```python
from build123d import *

# Parameters (mm, degrees)
SKETCH4_R           = 5
BOSS_EXTRUDE6_DEPTH = 15
SKETCH9_R           = 10.43494917
SKETCH9_R_2         = 5
BOSS_EXTRUDE8_DEPTH = 10.5


with BuildPart() as part:
    # Sketch4 → Boss-Extrude6 (new body)
    with BuildSketch(Plane.XY):
        with BuildLine():
            Line((101.689180826, -7.145205758), (62.319180826, -7.145205758))
            Line((62.319180826, -7.145205758), (62.319180826, 3.125413503))
            Line((62.319180826, 3.125413503), (101.689180826, 3.125413503))
            ThreePointArc((101.689180826, 3.125413503), (120.269891461, -2.009896128), (101.689180826, -7.145205758))
        make_face()
        with Locations((110.269891461, -2.009896128)):
            Circle(SKETCH4_R, mode=Mode.SUBTRACT)
    extrude(amount=BOSS_EXTRUDE6_DEPTH)

    # Sketch9 → Boss-Extrude8 (add)
    with BuildSketch(Plane(origin=(0, 3.125413503, 0), x_dir=(1, 0, 0), z_dir=(0, 1, 0))):
        with Locations(Location((55.063964483, -7.5, 0), (0, 0, 180))):
            Circle(SKETCH9_R)
        with Locations(Location((55.063964483, -7.5, 0), (0, 0, 180))):
            Circle(SKETCH9_R_2, mode=Mode.SUBTRACT)
    extrude(amount=-BOSS_EXTRUDE8_DEPTH)


solid = part.part
```
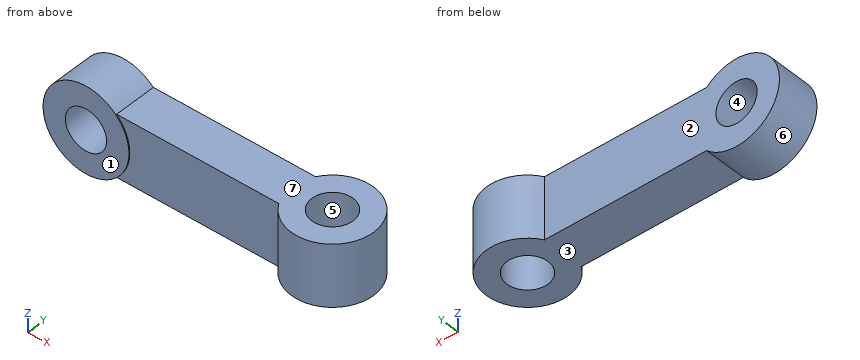
Input: part model. Units: mm. Frame: model coordinates. Face numbers are marked on the shaded views. A direction names the side the tool comes from. Round coordinates to 2 decimals unless told otherwise and drop trailing zeros. Loops run counter-clockwise (first coordinate to the right, second up) from the corner with the lowest first, then second, coordinate; pieces in that order, holes last. Notation, with made-up numbers: (-3, 23.25) - (48, 23.25) arc R11 cw to (48, 31.25) - close; hole circle Ø10 at (24, 50). An arc over 180 degrees is marked (long way). One line per item, written item: value. Start each with the question number.
(1) Section A-A, the plane z = 7.5. Return loops of the section in (x, y).
(2) Section B-B, the plane x = 107. Return loops of the section in (y, z), plus the area to 3 significant figures.
(3) Section C-C, the plane z = 13.5. Return loops of the section in (x, y), plus the area to 3 significant figures.
(4) Access query for the marked faces 1, 2 and 3. Directions: +Z, -Z, +X, -X, +Y, -Y. A direction counts if a zero-diameter tool reaches every point of the face in a straight line with its end or side. Return the directions, or none.
(5) Ray query, line 1 (X direction, y = -1, z = 5); line 2 (X direction, y = 0.5, z = 11.75); line 3 (Y direction, x = 59.5, z = -1.25). Return the intervals inside material, ascending. Write a range as [from, to].
(6) Section D-D, the plane z = 4.25. Return loops of the section in (x, y), plus the area to 3 significant figures.
(7) Draft query along Z for the marked faces 4, 5, 6 and 7. Return one class per face: +Z half, -Z half, draft (parallel to the pull), parting line (faces both ways), or undercut.
(8) Contact query for flat-ended pins moving along their axis: P1, Ø6, axis at x = 103, z = 2, coming from the +Y side; P2, Ø10, axis at y = -4.5, z = -0.5, coming from the -X side; P3, Ø1, axis at y = -4, z = 6, coming from the +X side. Output: stop coordinate, or through.
Results below:
1. outline: (44.63, -7.37) - (50.06, -7.37) - (50.06, 3.13) - (44.63, 3.13) - close; (60.06, -7.37) - (65.5, -7.37) - (65.5, -7.15) - (101.69, -7.15) arc R10 ccw (long way) to (101.69, 3.13) - (60.06, 3.13) - close; hole circle Ø10 at (110.27, -2.01)
2. outline: (-11.46, 0) - (-5.79, 0) - (-5.79, 15) - (-11.46, 15) - close; (1.77, 0) - (7.44, 0) - (7.44, 15) - (1.77, 15) - close
2. area: 170 mm^2
3. outline: (46.53, -7.37) - (63.6, -7.37) - (63.6, -7.15) - (101.69, -7.15) arc R10 ccw (long way) to (101.69, 3.13) - (46.53, 3.13) - close; hole circle Ø10 at (110.27, -2.01)
3. area: 796 mm^2
4. face 1: +Z, -Z, -X, -Y
4. face 2: +Z, -Z, -X, +Y
4. face 3: -Z, +X, +Y, -Y
5. line 1: [44.93, 50.73], [59.39, 105.37], [115.17, 120.22]
5. line 2: [45.53, 52.43], [57.7, 105.95], [114.59, 119.95]
5. line 3: [-7.37, 3.13]
6. outline: (45.15, -7.37) - (51.26, -7.37) - (51.26, 3.13) - (45.15, 3.13) - close; (58.86, -7.37) - (64.98, -7.37) - (64.98, -7.15) - (101.69, -7.15) arc R10 ccw (long way) to (101.69, 3.13) - (58.86, 3.13) - close; hole circle Ø10 at (110.27, -2.01)
6. area: 731 mm^2
7. face 4: undercut
7. face 5: draft
7. face 6: parting line
7. face 7: +Z half
8. P1: y = 7.03
8. P2: x = 45.07
8. P3: x = 120.16
